The listing builds one solid part. Answer for the finished solid, in the listing's coordinates (mm). Face numbers are marked on the shaded views. A direction names the side the tool comes from. Coordinates: 2 decimals unless noted, no trailing zeros. Loops run counter-clockwise (first coordinate to the right, second up) from the corner with the lowest first, then second, coordinate; pieces in that order, holes last. Notation, with made-up numbers: M 28.5,46 L 81.5,46 A29 cw 81.5,75 Z; hole C -14,7.25 d10. An arc over 180 degrees is marked long. Return JSON: item names as keys, results as strings. Group by question number.
1. Given P1, Ø5, axis at x = 138.5, y = 603.5, coming from the +Z side; P2, Ø12, axis at x = -68.5, y = 232.5, coming from the +Z side, each flat-ended and moving along its own axis, determine where each tip first touches the part or whether it passes through.
2. Section C-C (x = 153) is taken. Write down the section's boundary in (y, z).
3. Which of the six approach directions +Z, -Z, +X, -X, +Y, -Y give full straight-line access (tool end or side, diameter ignored) to the marked faces 1 and 2?
4. Section B-B (y = 201.5) is taken. Write down the section's boundary in (x, z), then the cut area to 3 significant figures.
5. Straight lines are drawn through the part: L1, parallel to X at y = 444, z = 33; L2, parallel to Y at x = 0, z = 31.5; L3, parallel to Y at x = 0, z = 36. For each, find the intervals that lie inside material, in ascending order. Write a range as from..to.
6. Section D-D (y = 732.5) is taken. Write down the section's boundary in (x, z), then the cut area to 3 significant figures.
7. The mould has two halves that part along Z. Classify the marked faces 3, 4 and 5: pulls with the +Z half, pulls with the -Z half, needs draft (parallel to the pull), parting line crosses it, or undercut.
8. Section A-A (x = 0) is taken. Write down the section's boundary in (y, z).
```python
from build123d import *

# Parameters (mm, degrees)
F1_DEPTH    = 247.65
F2_R        = 127
F3_R        = 25.4
F4_R        = 60.96
F5_T1_DEPTH = 736.9542394832
F6_R        = 38.1
F7_DEPTH    = 132.08
F8_R        = 63.5
F9_DEPTH    = 111.76


# Not quite as in the source:
# - a fillet or chamfer that OpenCascade refuses, or shapes differently, is made with other operations: its cross-section is extruded or revolved along the edge and cut away or added


with BuildPart() as f1:
    # F0 (on Right) → F1 (new body, symmetric)
    with BuildSketch(Plane.YZ):
        Polygon((-67.451213715, 0), (0, 0), (1270, 0), (1270, 48.26), (0, 48.26), (483.1377793135, 531.3977793135), (449.0128060535, 565.5227525736), (0, 116.5099465201), (-67.451213715, 49.0587328052), align=None)
    extrude(amount=F1_DEPTH, both=True)

    # F2
    f2_edges = [f1.edges().sort_by_distance(p)[0] for p in [
        (247.65, 466.075293, 548.460266),
        (-247.65, 466.075293, 548.460266),
        (247.65, 1270, 24.13),
        (-247.65, 1270, 24.13),
    ]]
    fillet(f2_edges, radius=F2_R)

    # F3
    f3_edges = [f1.edges().sort_by_distance(p)[0] for p in [
        (0, 0, 48.26),
    ]]
    fillet(f3_edges, radius=F3_R)

    # F4
    f4_edges = [f1.edges().sort_by_distance(p)[0] for p in [
        (0, -67.451214, 49.058733),
    ]]
    fillet(f4_edges, radius=F4_R)

    # F5: fillet of radius 60.96 on 1 edges, made by hand

    # F5_s2 → F5_t1 (cut)
    with BuildSketch(Plane.YZ.offset(-368.4771197416)):
        with BuildLine():
            ThreePointArc((-67.451213715, 23.8082740429), (-46.0587435131, 6.2750349075), (-19.1203658183, 0))
            Line((-19.1203658183, 0), (-67.451213715, 0))
            Line((-67.451213715, 0), (-67.451213715, 23.8082740429))
        make_face()
    extrude(amount=F5_T1_DEPTH, mode=Mode.SUBTRACT)

    # F6 (on face) → F7 (cut)
    with BuildSketch(Plane(origin=(0, -58.2549732601, 58.2549732601), x_dir=(1, 0, 0), z_dir=(0, -0.7071067812, 0.7071067812))):
        with Locations((-133.35, 526.8849732601)):
            Circle(F6_R)
        with Locations((133.35, 526.8849732601)):
            Circle(F6_R)
    extrude(amount=-F7_DEPTH, mode=Mode.SUBTRACT)

    # F8 (on Top) → F9 (cut)
    with BuildSketch(Plane.XY):
        with Locations((0, 444.5)):
            Circle(F8_R)
        with BuildLine():
            Line((-63.5, 838.2), (63.5, 838.2))
            ThreePointArc((63.5, 838.2), (0, 901.7), (-63.5, 838.2))
        make_face()
        with BuildLine():
            ThreePointArc((-63.5, 838.2), (0, 774.7), (63.5, 838.2))
            Line((63.5, 838.2), (-63.5, 838.2))
        make_face()
        with BuildLine():
            ThreePointArc((-63.5, 838.2), (0, 901.7), (63.5, 838.2))
            Line((63.5, 838.2), (63.5, 1092.2))
            ThreePointArc((63.5, 1092.2), (0, 1028.7), (-63.5, 1092.2))
            Line((-63.5, 1092.2), (-63.5, 838.2))
        make_face()
        with BuildLine():
            Line((-63.5, 1092.2), (63.5, 1092.2))
            ThreePointArc((63.5, 1092.2), (0, 1155.7), (-63.5, 1092.2))
        make_face()
        with BuildLine():
            ThreePointArc((-63.5, 1092.2), (0, 1028.7), (63.5, 1092.2))
            Line((63.5, 1092.2), (-63.5, 1092.2))
        make_face()
    extrude(amount=F9_DEPTH, mode=Mode.SUBTRACT)


solid = f1.part
```
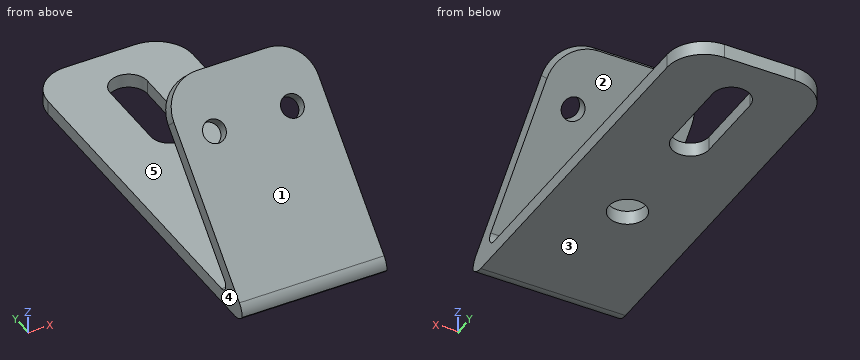
Worked out:
{
 "1": {"P1": "z = 48.26", "P2": "z = 355.01"},
 "2": {"outline": "M -67.45,23.81 A60.96 ccw -19.12,0 L 1265.81,0 L 1265.81,48.26 L 61.32,48.26 A25.4 cw 43.36,91.62 L 325.35,373.61 L 291.23,407.74 L -49.6,66.91 A60.96 ccw Z; M 337.39,453.9 L 371.52,419.78 L 480.18,528.44 L 446.05,562.56 Z"},
 "3": {"face 1": "+Z, +X, -X, -Y", "face 2": "+X, -X, +Y"},
 "4": {"outline": "M -247.65,0 L 247.65,0 L 247.65,48.26 L -247.65,48.26 Z; M -247.65,249.76 L 247.65,249.76 L 247.65,318.01 L -247.65,318.01 Z", "area": "57,700 mm^2"},
 "5": {"L1": "-247.65..-63.5, 63.5..247.65", "L2": "-66.96..381, 508..774.7, 1155.7..1270", "L3": "-66.22..381, 508..774.7, 1155.7..1270"},
 "6": {"outline": "M -247.65,0 L 247.65,0 L 247.65,48.26 L -247.65,48.26 Z", "area": "23,900 mm^2"},
 "7": {"face 3": "pulls with the -Z half", "face 4": "needs draft", "face 5": "undercut"},
 "8": {"outline": "M -67.45,23.81 A60.96 ccw -19.12,0 L 381,0 L 381,48.26 L 61.32,48.26 A25.4 cw 43.36,91.62 L 483.14,531.4 L 449.01,565.52 L -49.6,66.91 A60.96 ccw Z; M 508,0 L 774.7,0 L 774.7,48.26 L 508,48.26 Z; M 1155.7,0 L 1270,0 L 1270,48.26 L 1155.7,48.26 Z"}
}
